from build123d import *

# Parameters (mm, degrees)
F0_R     = 43.826874
F1_DEPTH = 25.4
F2_W     = 31.924735
F2_H     = 33.95685
F3_DEPTH = 25.4


with BuildPart() as f1:
    # F0 (on Front) → F1 (new body)
    with BuildSketch(Plane.XZ):
        with Locations((-22.304947, 20.578112)):
            Circle(F0_R)
    extrude(amount=F1_DEPTH)

    # F2 (on face) → F3 (cut)
    with BuildSketch(Plane.XZ.offset(25.4)):
        with Locations((-22.304946, 20.578112)):
            Rectangle(F2_W, F2_H)
    extrude(amount=-F3_DEPTH, mode=Mode.SUBTRACT)


solid = f1.part
Here's how the part is built. I have some questions about the finished solid (model axes, mm). A direction names the side the tool comes from. Give positions to 0.01 mm unless a question says otherwise; leave off trailing zeros. Write each loop counter-clockwise with the first axis right and the second up, starting at its lowest first coordinate (ties: lowest second). Pieces come first, ordered by that corner, then holes. Notation, with made-up numbers: (-36.75, 27.25) -> (-29.75, 27.25) arc R10 cw to (-29.75, 44.25) -> close; hole circle Ø3 at (20, -7.75). An arc over 180 degrees is marked (long way). Use one line per item in the form item = value. Start each with the question number.
1. If I drill on L1, parallel to X at y = -15, z = 22; L2, parallel to Z at x = -23.5, y = -10; L3, parallel to Z at x = -31, y = -20, over which ranges is the centre line in solid material (lowest first)?
2. Imagine slicing it at A-A on x = -17. List the corners of the cut face in (y, z) for me.
3. Thinking about a two-plate mould opening in Z: for faces 3 (the face through (-23, -13, 37.557)), 4 (the face through (19.5, -12.52, 33.74)), 5 (the face through (-23, 0, 2)), 6 (the face through (-38.267, -13, 20)), which applies, +Z half, -Z half, draft (parallel to the pull), parting line (faces both ways), or undercut?
4. Imagine slicing it at B-B on z = 8.5. List the corners of the cut face in (x, y) for me, plus the area to 3 significant figures.
5. Imagine slicing it at C-C on y = -8. List the corners of the cut face in (x, z) for me.
6. On a 3-axis mill with a long thin cutter (end or side, diameter ignored), from which of +Z, -Z, +X, -X, +Y, -Y can I reach the whole of each face in a straight line? I mean faces 1 (the face through (-23, -25.4, 2)), 2 (the face through (-23, -13, 3.6)). Say none if no direction works.
7. Imagine slicing it at D-D on x = -42. List the corners of the cut face in (y, z) for me, plus the area to 3 significant figures.
8. Will these pins go through, and if not, where does the flat tip stop? pin 1 Ø6 at (y, z) = (-12.5, 38.5) entering from +X; pin 2 Ø1.5 at (x, y) = (-39.5, -4) entering from +Z; pin 3 Ø12 at (x, y) = (-37.5, -14) entering from -Z; pin 4 Ø3 at (y, z) = (-2.5, 20) entering from +X.
Entries:
q1.L1 = -66.11 to -38.27, -6.34 to 21.5
q1.L2 = -23.23 to 3.6, 37.56 to 64.39
q1.L3 = -22.38 to 3.6, 37.56 to 63.53
q2.outline = (-25.4, -22.93) -> (0, -22.93) -> (0, 3.6) -> (-25.4, 3.6) -> close; (-25.4, 37.56) -> (0, 37.56) -> (0, 64.08) -> (-25.4, 64.08) -> close
q3.face_3 = undercut
q3.face_4 = parting line
q3.face_5 = draft
q3.face_6 = undercut
q4.outline = (-64.43, -25.4) -> (-38.27, -25.4) -> (-38.27, 0) -> (-64.43, 0) -> close; (-6.34, -25.4) -> (19.82, -25.4) -> (19.82, 0) -> (-6.34, 0) -> close
q4.area = 1,330 mm²
q5.outline = circle Ø87.65 at (-22.3, 20.58); hole (-38.27, 3.6) -> (-6.34, 3.6) -> (-6.34, 37.56) -> (-38.27, 37.56) -> close
q6.face_1 = +Z, -Z, +X, -X, -Y
q6.face_2 = +Y, -Y
q7.outline = (-25.4, -18.57) -> (0, -18.57) -> (0, 59.73) -> (-25.4, 59.73) -> close
q7.area = 1,990 mm²
q8.pin_1 = 18.9
q8.pin_2 = 61.2
q8.pin_3 = -22.27
q8.pin_4 = 21.52
